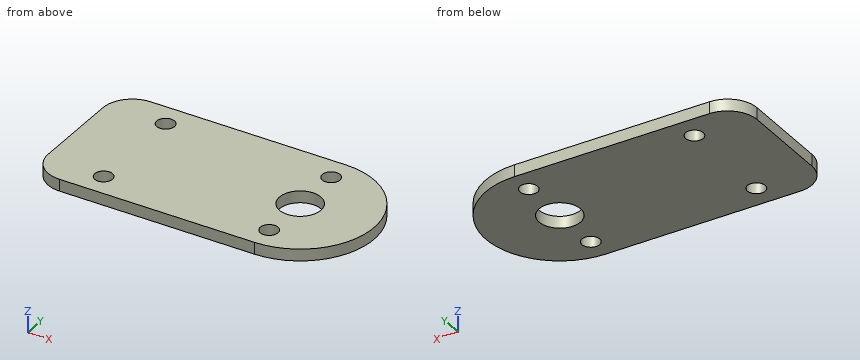
from build123d import *

# Parameters (mm, degrees)
SKETCH_1_R      = 3.5
SKETCH_1_R_2    = 1.5
EXTRUDE_1_DEPTH = 2
FILLET_1_R      = 5


with BuildPart() as part:
    # 草图1 → 凸台-拉伸1 (new body)
    with BuildSketch(Plane.XY):
        with BuildLine():
            Line((21.5, -12.5), (-16.5, -12.5))
            Line((-16.5, -12.5), (-16.5, 12.5))
            Line((-16.5, 12.5), (21.5, 12.5))
            ThreePointArc((21.5, 12.5), (34, 0), (21.5, -12.5))
        make_face()
        with Locations((21.5, 0)):
            Circle(SKETCH_1_R, mode=Mode.SUBTRACT)
        with Locations((21.5, 8.5)):
            Circle(SKETCH_1_R_2, mode=Mode.SUBTRACT)
        with Locations(Location((21.5, -8.5, 0), (0, 0, 180))):
            Circle(SKETCH_1_R_2, mode=Mode.SUBTRACT)
        with Locations((-6.5, 8.5)):
            Circle(SKETCH_1_R_2, mode=Mode.SUBTRACT)
        with Locations(Location((-6.5, -8.5, 0), (0, 0, 180))):
            Circle(SKETCH_1_R_2, mode=Mode.SUBTRACT)
    extrude(amount=EXTRUDE_1_DEPTH)

    # 圆角1
    fillet_1_edges = [part.edges().sort_by_distance(p)[0] for p in [
        (-16.5, 12.5, 1),
        (-16.5, -12.5, 1),
    ]]
    fillet(fillet_1_edges, radius=FILLET_1_R)


solid = part.part
Work out the finished part from the listing and answer in its coordinate system (mm). Coordinates: 2 decimals unless noted, no trailing zeros. Loops run counter-clockwise (first coordinate to the right, second up) from the corner with the lowest first, then second, coordinate; pieces in that order, holes last. Notation, with made-up numbers: (-8.75, -15.5) -> (4.25, -15.5) arc R26 ccw to (4.25, 20.5) -> close; hole circle Ø3 at (7.25, -11). An arc over 180 degrees is marked (long way). Write each question's results on one line, items separated by ' | '. Start each with the question number.
1) Find section C-C on z = 0.45. Determine the outline of the cut face in (x, y).
2) Find section D-D on y = 8.5. Determine the outline of the cut face in (x, z), then the cut area to 3 significant figures.
3) Consider line 1 along Y through (x, z) = (-6.5, 0.85); line 2 along Y through (x, z) = (21.5, 1.1); line 3 along X through (y, z) = (0.25, 1.85). Determine where each line is inside the solid, lowest interval first.
4) Flat-ended cylindrical pins translate along their axes: P1, Ø4, axis at x = 21.5, y = 0, coming from the -Z side; P2, Ø2, axis at x = 13, y = -7.5, coming from the -Z side. Find the tip coordinate at first contact, or state that the pin passes through.
5) Find section B-B on x = -6.5. Determine the outline of the cut face in (y, z).
6) Find section A-A on y = 0. Determine the outline of the cut face in (x, z), then the cut area to 3 significant figures.
Response values:
1) outline: (-16.5, -7.5) arc R5 ccw to (-11.5, -12.5) -> (21.5, -12.5) arc R12.5 ccw to (21.5, 12.5) -> (-11.5, 12.5) arc R5 ccw to (-16.5, 7.5) -> close; hole circle Ø3 at (-6.5, -8.5); hole circle Ø3 at (-6.5, 8.5); hole circle Ø7 at (21.5, 0); hole circle Ø3 at (21.5, -8.5); hole circle Ø3 at (21.5, 8.5)
2) outline: (-16.4, 0) -> (-8, 0) -> (-8, 2) -> (-16.4, 2) -> close; (-5, 0) -> (20, 0) -> (20, 2) -> (-5, 2) -> close; (23, 0) -> (30.67, 0) -> (30.67, 2) -> (23, 2) -> close | area: 82.1 mm^2
3) line 1: y = -12.5 to -10, -7 to 7, 10 to 12.5 | line 2: y = -12.5 to -10, -7 to -3.5, 3.5 to 7, 10 to 12.5 | line 3: x = -16.5 to 18.01, 24.99 to 34
4) P1: passes through | P2: stops at z = 0
5) outline: (-12.5, 0) -> (-10, 0) -> (-10, 2) -> (-12.5, 2) -> close; (-7, 0) -> (7, 0) -> (7, 2) -> (-7, 2) -> close; (10, 0) -> (12.5, 0) -> (12.5, 2) -> (10, 2) -> close
6) outline: (-16.5, 0) -> (18, 0) -> (18, 2) -> (-16.5, 2) -> close; (25, 0) -> (34, 0) -> (34, 2) -> (25, 2) -> close | area: 87.0 mm^2
